from build123d import *

# Parameters (mm, degrees)
F2_R     = 5.08
F3_DEPTH = 20.32
F5_DEPTH = 15.24
F7_DEPTH = 15.24


with BuildPart() as f1:
    # F0 (on Front) → F1 (revolve)
    with BuildSketch(Plane.XZ):
        Polygon((-22.86, 0), (0, 0), (0, 50.8), (0, 63.5), (0, 109.22), (-7.62, 109.22), (-7.62, 127), (-12.7, 127), (-12.7, 63.5), (-12.7, 50.8), (-22.86, 20.32), align=None)
    revolve(axis=Axis((0, 0, 86.36), (0, 0, -1)))

    # F2 (on Top) → F3 (cut)
    with BuildSketch(Plane.XY):
        with BuildLine():
            ThreePointArc((5.08, 10.16), (-3.592102, 13.752102), (0, 5.08))
            ThreePointArc((0, 5.08), (3.592102, 6.567898), (5.08, 10.16))
        make_face()
        with BuildLine():
            ThreePointArc((15.24, 0), (10.16, 5.08), (5.08, 0))
            ThreePointArc((5.08, 0), (10.16, -5.08), (15.24, 0))
        make_face()
        with BuildLine():
            ThreePointArc((5.08, -10.245183), (3.592102, -6.65308), (0, -5.165183))
            ThreePointArc((0, -5.165183), (-3.592102, -13.837285), (5.08, -10.245183))
        make_face()
        with Locations((-10.16, 0)):
            Circle(F2_R)
    extrude(amount=F3_DEPTH, mode=Mode.SUBTRACT)

    # F4 (on Right) → F5 (cut, symmetric)
    with BuildSketch(Plane.YZ):
        Polygon((-2.54, 63.5), (0, 63.5), (2.54, 63.5), (2.54, 101.6), (-2.54, 101.6), align=None)
    extrude(amount=F5_DEPTH, both=True, mode=Mode.SUBTRACT)

    # F6 (on Front) → F7 (cut, symmetric)
    with BuildSketch(Plane.XZ):
        Polygon((-2.54, 63.5), (0, 63.5), (2.54, 63.5), (2.54, 101.6), (-2.54, 101.6), align=None)
    extrude(amount=F7_DEPTH, both=True, mode=Mode.SUBTRACT)


solid = f1.part
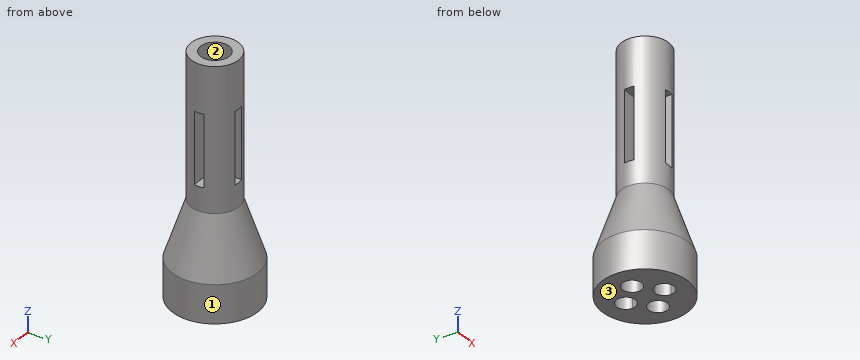
The listing builds one solid part. Answer for the finished solid, in the listing's coordinates (mm). Face numbers are marked on the shaded views. Give positions to 0.01 mm unless a question says otherwise; leave off trailing zeros. Loops run counter-clockwise (first coordinate to the right, second up) from the corner with the lowest first, then second, coordinate; pieces in that order, holes last. Notation, with made-up numbers: (25.25, -35) - (68.25, -35) arc R11 cw to (68.25, -29) - close; hole circle Ø6 at (4.25, -26.75). An arc over 180 degrees is marked (long way). Write each question's results on one line, items separated by ' | '.
1. Find section C-C, the plane z = 33. Write down the section's boundary in (x, y).
Resolved:
outline: circle Ø37.27 at (0, 0)
2. Flat-ended cylindrical pins translate along their axes: P1, Ø3, axis at y = -8, z = 91, coming from the -X side; P2, Ø3, axis at x = 5.5, z = 81, coming from the -Y side; P3, Ø12, axis at y = 6, z = 105.5, coming from the +X side; P4, Ø6, axis at y = 17.5, z = 90, coming from the -X side (1 decimal). Find the tip coordinate at first contact, or state that the pin passes through.
Resolved:
P1: stops at x = -10.91 | P2: stops at y = -12.05 | P3: stops at x = 12.7 | P4: passes through
3. Find section A-A, the plane y = 0. Write down the section's boundary in (x, z), then the cut area to 3 significant figures.
Resolved:
outline: (-22.86, 0) - (-15.24, 0) - (-15.24, 20.32) - (-5.08, 20.32) - (-5.08, 0) - (5.08, 0) - (5.08, 20.32) - (15.24, 20.32) - (15.24, 0) - (22.86, 0) - (22.86, 20.32) - (12.7, 50.8) - (12.7, 63.5) - (-12.7, 63.5) - (-12.7, 50.8) - (-22.86, 20.32) - close; (-12.7, 101.6) - (12.7, 101.6) - (12.7, 127) - (7.62, 127) - (7.62, 109.22) - (-7.62, 109.22) - (-7.62, 127) - (-12.7, 127) - close | area: 2,300 mm^2
4. Consider probe 1 along Y at (x, z) = (0, 121); probe 2 along Y at (x, z) = (-3.5, 86); probe 3 along X at (y, z) = (-8, 69). Determine where each line is inside the solid, lowest interval first. Write a range as from..to.
Resolved:
probe 1: y = -12.7..-7.62, 7.62..12.7 | probe 2: y = -12.21..-2.54, 2.54..12.21 | probe 3: x = -9.86..-2.54, 2.54..9.86
5. Find section B-B, the plane z = 67.5. Write down the section's boundary in (x, y).
Resolved:
outline: (-12.44, -2.54) arc R12.7 ccw to (-2.54, -12.44) - (-2.54, -2.54) - close; (-12.44, 2.54) - (-2.54, 2.54) - (-2.54, 12.44) arc R12.7 ccw to start; (2.54, -12.44) arc R12.7 ccw to (12.44, -2.54) - (2.54, -2.54) - close; (2.54, 2.54) - (12.44, 2.54) arc R12.7 ccw to (2.54, 12.44) - close
6. For a pull along X with two mould halves and no side action, classify the marked faces 1, 2 and 3 as +X half, -X half, draft (parallel to the pull), parting line (faces both ways), or undercut.
Resolved:
face 1: parting line | face 2: undercut | face 3: draft
